For this review, take the finished solid that the model builds, in its own axes (mm). Coordinates: 2 decimals unless noted, no trailing zeros. Loops run counter-clockwise (first coordinate to the right, second up) from the corner with the lowest first, then second, coordinate; pieces in that order, holes last.
1. Take a section at C-C, the plane z = 32. State the section outline as (x, y) points, then the cut area to 3 significant figures.
2. Take a section at A-A, the plane x = -25.4. State the section outline as (y, z) points.
3. Clearance check with flat-ended pins moving along their axes: P1, Ø3, axis at x = -17.5, z = 60.5, coming from the -Y side; P2, Ø2, axis at x = -40, z = 49, coming from the +Y side; P3, Ø12, axis at x = -20, z = 45, coming from the -Y side. State where each tip first meets the part, or that it passes through.
4. Take a section at D-D, the plane z = 61. State the section outline as (x, y) points.
5. To check wall thickness, follow probe 1 along Z at (x, y) = (-46.5, 12); probe 2 along Z at (x, y) = (-5.5, -15); probe 3 along Y at (x, z) = (-2.5, 56). State the ranges of each line that lie inside material, in increasing order.
6. Take a section at B-B, the plane y = 0. State the section outline as (x, z) points.
```python
from build123d import *

# Parameters (mm, degrees)
F2_R    = 5.08
F3_SIZE = 5.08


with BuildPart() as f1:
    # F0 (on Front) → F1 (revolve)
    with BuildSketch(Plane.XZ):
        with BuildLine():
            Line((-25.4, 0), (0, 0))
            Line((0, 0), (0, 10.6707542909))
            ThreePointArc((0, 10.6707542909), (-4.6695087331, 15.340263024), (0, 20.0097717571))
            Line((0, 20.0097717571), (0, 56.8024416143))
            ThreePointArc((0, 56.8024416143), (-4.8593978709, 61.6618394852), (0, 66.521237356))
            Line((0, 66.521237356), (0, 76.2))
            Line((0, 76.2), (-25.4, 76.2))
            Line((-25.4, 76.2), (-25.4, 0))
        make_face()
    revolve(axis=Axis((-25.4, 0, 38.1), (0, 0, 1)))

    # F2
    f2_edges = [f1.edges().sort_by_distance(p)[0] for p in [
        (-50.8, 0, 76.2),
    ]]
    fillet(f2_edges, radius=F2_R)

    # F3
    f3_edges = [f1.edges().sort_by_distance(p)[0] for p in [
        (-50.8, 0, 0),
    ]]
    chamfer(f3_edges, length=F3_SIZE)


solid = f1.part
```
Results list:
1. outline: circle Ø50.8 at (-25.4, 0)
1. area: 2,030 mm2
2. outline: (-25.4, 5.08) - (-20.32, 0) - (20.32, 0) - (25.4, 5.08) - (25.4, 10.67) arc R4.67 cw to (25.4, 20.01) - (25.4, 56.8) arc R4.86 cw to (25.4, 66.52) - (25.4, 71.12) arc R5.08 ccw to (20.32, 76.2) - (-20.32, 76.2) arc R5.08 ccw to (-25.4, 71.12) - (-25.4, 66.52) arc R4.86 cw to (-25.4, 56.8) - (-25.4, 20.01) arc R4.67 cw to (-25.4, 10.67) - close
3. P1: stops at y = -19.97
3. P2: stops at y = 21.45
3. P3: stops at y = -25.4
4. outline: circle Ø41.17 at (-25.4, 0)
5. probe 1: z = 3.95 to 10.81, 19.87 to 56.93, 66.39 to 74.31
5. probe 2: z = 4.6 to 10.7, 19.99 to 56.83, 66.5 to 73.28
5. probe 3: y = -10.99 to 10.99
6. outline: (-50.8, 5.08) - (-45.72, 0) - (-5.08, 0) - (0, 5.08) - (0, 10.67) arc R4.67 cw to (0, 20.01) - (0, 56.8) arc R4.86 cw to (0, 66.52) - (0, 71.12) arc R5.08 ccw to (-5.08, 76.2) - (-45.72, 76.2) arc R5.08 ccw to (-50.8, 71.12) - (-50.8, 66.52) arc R4.86 cw to (-50.8, 56.8) - (-50.8, 20.01) arc R4.67 cw to (-50.8, 10.67) - close
